from build123d import *

# Parameters (mm, degrees)
SKETCH1_W           = 50.8
SKETCH1_H           = 127
SKETCH1_R           = 9.525
SKETCH1_R_2         = 6.35
BOSS_EXTRUDE1_DEPTH = 6.35
SKETCH2_R           = 1.778
CUT_EXTRUDE1_DEPTH  = 6.35
CIRPATTERN1_COUNT   = 4
SKETCH3_R           = 1.778
CUT_EXTRUDE2_DEPTH  = 6.35
CIRPATTERN2_COUNT   = 8
FILLET1_R           = 6.35


with BuildPart() as part:
    # Sketch1 → Boss-Extrude1 (new body)
    with BuildSketch(Plane.XY):
        with Locations((25.4, 63.5)):
            Rectangle(SKETCH1_W, SKETCH1_H)
        with Locations((25.4, 25.4)):
            Circle(SKETCH1_R, mode=Mode.SUBTRACT)
        with Locations((25.4, 107.95)):
            Circle(SKETCH1_R_2, mode=Mode.SUBTRACT)
    extrude(amount=BOSS_EXTRUDE1_DEPTH)

    # Sketch2 → Cut-Extrude1 (cut)
    with BuildSketch(Plane.XY.offset(6.35)):
        with Locations((25.4, 44.45)):
            Circle(SKETCH2_R)
    cut_extrude1 = extrude(amount=-CUT_EXTRUDE1_DEPTH, mode=Mode.SUBTRACT)

    # CirPattern1: Cut-Extrude1 ×4 about axis
    cirpattern1_axis = Axis((25.4, 25.4, 0), (0, 0, 1))
    for i in range(1, CIRPATTERN1_COUNT):
        add(cut_extrude1.rotate(cirpattern1_axis, i * 360 / CIRPATTERN1_COUNT), mode=Mode.SUBTRACT)

    # Sketch3 → Cut-Extrude2 (cut)
    with BuildSketch(Plane.XY.offset(6.35)):
        with Locations((25.4, 117.729)):
            Circle(SKETCH3_R)
    cut_extrude2 = extrude(amount=-CUT_EXTRUDE2_DEPTH, mode=Mode.SUBTRACT)

    # CirPattern2: Cut-Extrude2 ×8 about axis
    cirpattern2_axis = Axis((25.4, 107.95, 0), (0, 0, 1))
    for i in range(1, CIRPATTERN2_COUNT):
        add(cut_extrude2.rotate(cirpattern2_axis, i * 360 / CIRPATTERN2_COUNT), mode=Mode.SUBTRACT)

    # Fillet1
    fillet1_edges = [part.edges().sort_by_distance(p)[0] for p in [
        (0, 127, 3.175),
        (50.8, 127, 3.175),
        (50.8, 0, 3.175),
        (0, 0, 3.175),
    ]]
    fillet(fillet1_edges, radius=FILLET1_R)


solid = part.part
Here's how the part is built. I have some questions about the finished solid (model axes, mm). Round coordinates to 2 decimals unless told otherwise and drop trailing zeros. Loops run counter-clockwise (first coordinate to the right, second up) from the corner with the lowest first, then second, coordinate; pieces in that order, holes last. Notation, with made-up numbers: (23.5, 87.5) -> (71.5, 87.5) arc R24 ccw to (71.5, 100.5) -> close; hole circle Ø3 at (-20.5, 40.25). An arc over 180 degrees is marked (long way). Write each question's results on one line, items separated by ' | '.
(1) If we section it at B-B, the plane x = 25.4: List the corners of the cut face in (y, z) for me (3 decimals).
Worked answers:
outline: (0, 0) -> (4.572, 0) -> (4.572, 6.35) -> (0, 6.35) -> close; (8.128, 0) -> (15.875, 0) -> (15.875, 6.35) -> (8.128, 6.35) -> close; (34.925, 0) -> (42.672, 0) -> (42.672, 6.35) -> (34.925, 6.35) -> close; (46.228, 0) -> (96.393, 0) -> (96.393, 6.35) -> (46.228, 6.35) -> close; (99.949, 0) -> (101.6, 0) -> (101.6, 6.35) -> (99.949, 6.35) -> close; (114.3, 0) -> (115.951, 0) -> (115.951, 6.35) -> (114.3, 6.35) -> close; (119.507, 0) -> (127, 0) -> (127, 6.35) -> (119.507, 6.35) -> close
(2) If we section it at D-D, the plane z = 1.5: Give the number of separate pieces and of enclosed holes in the cut face, then the cut area to 3 significant figures.
Worked answers:
separate pieces: 1 | enclosed holes: 14 | area: 5,890 mm2
(3) If I drill on L1, parallel to X at y = 6.35, z = 3; L2, parallel to Y at x = 19, z = 1; L3, parallel to Y at x = 6.5, z = 0.5, over which ranges is the centre line in solid material (lowest first)?
Worked answers:
L1: 0 to 23.62, 27.18 to 50.8 | L2: 0 to 18.35, 32.45 to 99.33, 102.74 to 113.16, 116.57 to 127 | L3: 0 to 23.63, 27.17 to 127
(4) If we section it at A-A, the plane y = 44.45: List the corners of the cut face in (x, z) for me.
Worked answers:
outline: (0, 0) -> (23.62, 0) -> (23.62, 6.35) -> (0, 6.35) -> close; (27.18, 0) -> (50.8, 0) -> (50.8, 6.35) -> (27.18, 6.35) -> close
(5) We'd pull the mould along X, two halves only. Please class faces 1 (the face through (27.176, 6.272, 3.219)), 2 (the face through (1.81, 125.09, 3.22)), 3 (the face through (48.89, 125.19, 3.22)), 4 (the face through (32.99, 113.22, 3.22)): released by +X, released by -X, zero draft, split by the parting line, or undercut.
Worked answers:
face 1: undercut | face 2: released by -X | face 3: released by +X | face 4: undercut
(6) If we section it at C-C, the plane y = 107.95: List the corners of the cut face in (x, z) for me.
Worked answers:
outline: (0, 0) -> (13.84, 0) -> (13.84, 6.35) -> (0, 6.35) -> close; (17.4, 0) -> (19.05, 0) -> (19.05, 6.35) -> (17.4, 6.35) -> close; (31.75, 0) -> (33.4, 0) -> (33.4, 6.35) -> (31.75, 6.35) -> close; (36.96, 0) -> (50.8, 0) -> (50.8, 6.35) -> (36.96, 6.35) -> close
